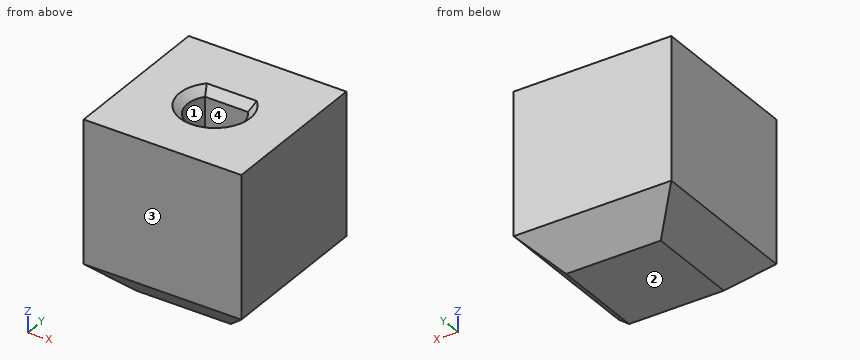
from build123d import *

# Parameters (mm, degrees)
BOX406008008_W     = 10
BOX406008008_H     = 10
BOX406008008_DEPTH = 19
CYLINDER079_R      = 1.75
CYLINDER079_DEPTH  = 17
BOX406008009_W     = 10
BOX406008009_H     = 10
BOX406008009_DEPTH = 11
CHAMFER004_SIZE    = 2
CHAMFER008_SIZE    = 0.5


with BuildPart() as cube343:
    # Box406008008 → Box406008008 (new body)
    with BuildSketch(Plane(origin=(-5, 1.1, 1.5), x_dir=(1, 0, 0), z_dir=(0, 0, 1))):
        with Locations((5, 5)):
            Rectangle(BOX406008008_W, BOX406008008_H)
    extrude(amount=BOX406008008_DEPTH)


with BuildPart() as motor_shaft_hole:
    # Cylinder079 → Cylinder079 (new body)
    with BuildSketch(Plane.XY.offset(9)):
        Circle(CYLINDER079_R)
    extrude(amount=CYLINDER079_DEPTH)

    # Cut064: cut Cube343
    add(cube343.part, mode=Mode.SUBTRACT)


with BuildPart() as chamfer008:
    # Box406008009 → Box406008009 (new body)
    with BuildSketch(Plane(origin=(-5, -5, 7), x_dir=(1, 0, 0), z_dir=(0, 0, 1))):
        with Locations((5, 5)):
            Rectangle(BOX406008009_W, BOX406008009_H)
    extrude(amount=BOX406008009_DEPTH)

    # Cut065: cut Motor Shaft Hole
    add(motor_shaft_hole.part, mode=Mode.SUBTRACT)

    # Chamfer004
    chamfer004_edges = [chamfer008.edges().sort_by_distance(p)[0] for p in [
        (-5, 0, 7),
        (0, -5, 7),
        (0, 5, 7),
        (5, 0, 7),
    ]]
    chamfer(chamfer004_edges, length=CHAMFER004_SIZE)

    # Chamfer008
    chamfer008_edges = [chamfer008.edges().sort_by_distance(p)[0] for p in [
        (1.649904, 0.583367, 18),
        (0, 1.1, 18),
        (-0.583367, -1.649904, 18),
    ]]
    chamfer(chamfer008_edges, length=CHAMFER008_SIZE)


solid = chamfer008.part
Work out the finished part from the listing and answer in its coordinate system (mm). Face numbers are marked on the shaded views. Give positions to 0.01 mm unless a question says otherwise; leave off trailing zeros. Order: outer loops, then holes, each group sorted by start corner. A loop starts at its lowest first (then second) coordinate and runs counter-clockwise, first axis right, second up. Notation, with made-up numbers: (38.5, -2.75) -> (81.5, -2.75) arc R37 cw to (81.5, 35.25) -> close; hole circle Ø10 at (36, 87.5). An arc over 180 degrees is marked (long way). Answer as a JSON object with one key per item and string values. Group by question number.
1. Section B-B on y = 0 is taken. Determine the outline of the cut face in (x, z), plus the area to 4 significant figures.
2. Consider line 1 along Y through (x, z) = (0, 13); line 2 along X through (y, z) = (0, 10); line 3 along X through (y, z) = (-1.5, 9.5). Determine where each line is inside the solid, lowest interval first. Write a range as [from, to].
3. Section D-D on x = 4.5 is taken. Determine the outline of the cut face in (y, z), plus the area to 4 significant figures.
4. A flat-ended cylindrical pin translates along its axis: pin 1 Ø2 at (x, y) = (0, 0) entering from +Z. Find the tip coordinate at first contact, or state that the pin passes through.
5. Section C-C on z = 17 is taken. Determine the outline of the cut face in (x, y).
6. Section A-A on x = 0 is taken. Determine the outline of the cut face in (y, z), plus the area to 3 significant figures.
7. The mould has two halves that part along Y. Classify the marked faces 1, 2, 3 and 4: released by +Y, released by -Y, zero draft, split by the parting line, or undercut.
Result sheet:
{
 "1": {"outline": "(-5, 9) -> (-3, 7) -> (3, 7) -> (5, 9) -> (5, 18) -> (2.25, 18) -> (1.75, 17.5) -> (1.75, 9) -> (-1.75, 9) -> (-1.75, 17.5) -> (-2.25, 18) -> (-5, 18) -> close", "area": "74.25 mm^2"},
 "2": {"line 1": "y = [-5, -1.75], [1.1, 5]", "line 2": "x = [-5, -1.75], [1.75, 5]", "line 3": "x = [-5, -0.9], [0.9, 5]"},
 "3": {"outline": "(-5, 9) -> (-4.5, 8.5) -> (4.5, 8.5) -> (5, 9) -> (5, 18) -> (-5, 18) -> close", "area": "94.75 mm^2"},
 "4": {"pin 1": "stops at z = 9"},
 "5": {"outline": "(-5, -5) -> (5, -5) -> (5, 5) -> (-5, 5) -> close; hole (-1.36, 1.1) arc R1.75 ccw (long way) to (1.36, 1.1) -> close"},
 "6": {"outline": "(-5, 9) -> (-3, 7) -> (3, 7) -> (5, 9) -> (5, 18) -> (1.6, 18) -> (1.1, 17.5) -> (1.1, 9) -> (-1.75, 9) -> (-1.75, 17.5) -> (-2.25, 18) -> (-5, 18) -> close", "area": "80.1 mm^2"},
 "7": {"face 1": "undercut", "face 2": "zero draft", "face 3": "released by -Y", "face 4": "undercut"}
}
